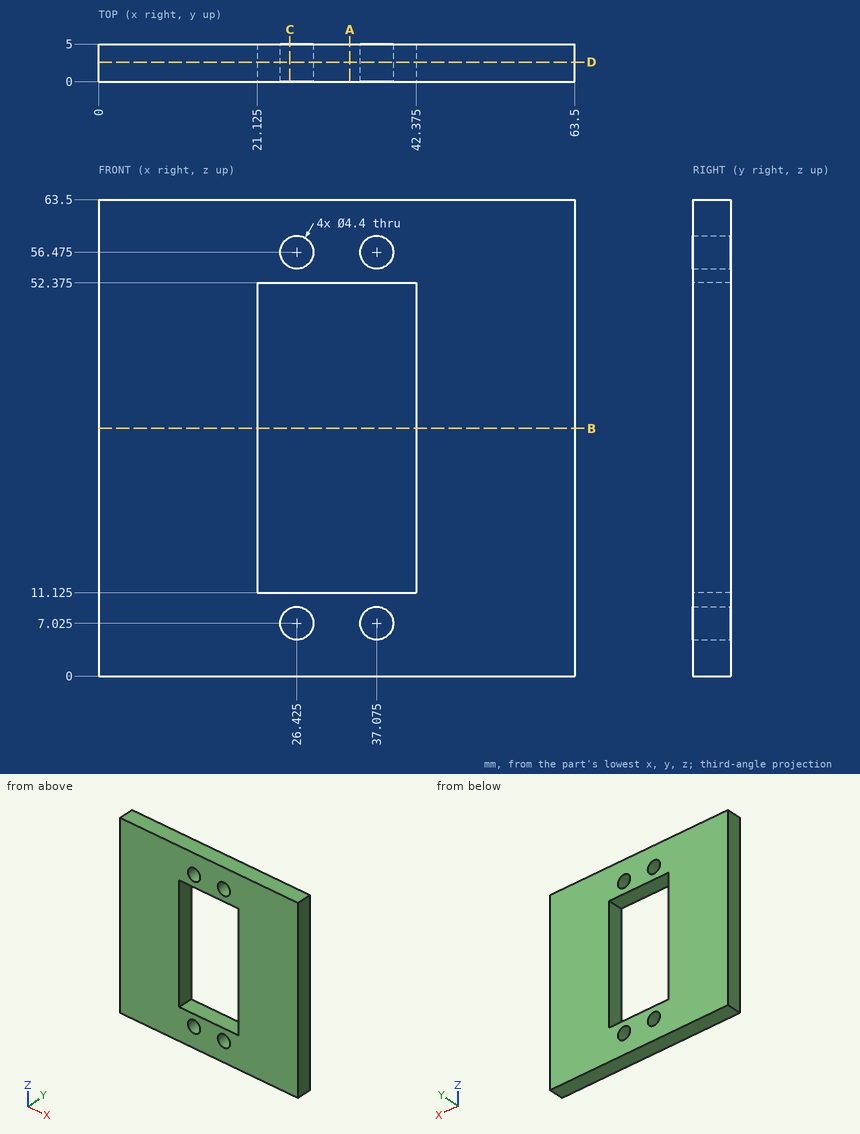
The drawing under review shows one solid part. Ordinate dimensions are in mm from its lowest x, y, z. Round coordinates to 2 decimals unless told otherwise and drop trailing zeros. Loops run counter-clockwise (first coordinate to the right, second up) from the corner with the lowest first, then second, coordinate; pieces in that order, holes last. Notation, with made-up numbers: (-18.75, 35.25) -> (4.25, 35.25) arc R34 ccw to (4.25, 65.25) -> close; hole circle Ø7 at (-20, 37.25). An arc over 180 degrees is marked (long way). One line per question, with ' | ' between items. Start each with the question number.
Item 1: Add section C-C, the plane x = 25.5. Write out the cut boundary in (y, z) (3 decimals).
Item 2: Wall thickness on line 1 along X through (y, z) = (0.8, 33.5) (3 decimals); line 2 along X through (y, z) = (3.6, 56); line 3 along Z through (x, y) = (21.5, 4.6) (3 decimals): over which ranges is each line inside the solid? List them lowest first. Write a range as [from, to].
Item 3: Add section A-A, the plane x = 33.5. Write out the cut boundary in (y, z) (3 decimals).
Item 4: Add section B-B, the plane z = 33. Write out the cut boundary in (x, y) (3 decimals).
Item 5: Add section D-D, the plane y = 2.6. Write out the cut boundary in (x, z) (3 decimals).
Return value:
1) outline: (0, 0) -> (5, 0) -> (5, 5.029) -> (0, 5.029) -> close; (0, 9.021) -> (5, 9.021) -> (5, 11.125) -> (0, 11.125) -> close; (0, 52.375) -> (5, 52.375) -> (5, 54.479) -> (0, 54.479) -> close; (0, 58.471) -> (5, 58.471) -> (5, 63.5) -> (0, 63.5) -> close
2) line 1: x = [0, 21.125], [42.375, 63.5] | line 2: x = [0, 24.28], [28.57, 34.93], [39.22, 63.5] | line 3: z = [0, 11.125], [52.375, 63.5]
3) outline: (0, 0) -> (5, 0) -> (5, 11.125) -> (0, 11.125) -> close; (0, 52.375) -> (5, 52.375) -> (5, 63.5) -> (0, 63.5) -> close
4) outline: (0, 0) -> (21.125, 0) -> (21.125, 5) -> (0, 5) -> close; (42.375, 0) -> (63.5, 0) -> (63.5, 5) -> (42.375, 5) -> close
5) outline: (0, 0) -> (63.5, 0) -> (63.5, 63.5) -> (0, 63.5) -> close; hole (21.125, 11.125) -> (42.375, 11.125) -> (42.375, 52.375) -> (21.125, 52.375) -> close; hole circle Ø4.4 at (26.425, 7.025); hole circle Ø4.4 at (26.425, 56.475); hole circle Ø4.4 at (37.075, 7.025); hole circle Ø4.4 at (37.075, 56.475)
